from build123d import *

# Parameters (mm, degrees)
SKETCH_1_W          = 37
SKETCH_1_H          = 37
EXTRUDE_1_DEPTH     = 10.5
SKETCH_2_R          = 10
CUT_EXTRUDE_1_DEPTH = 11.5
FILLET_1_R          = 5
FILLET_2_R          = 1
SKETCH_3_R          = 1.5
CUT_EXTRUDE_2_DEPTH = 4
CUT_EXTRUDE_3_DEPTH = 8.5
CUT_EXTRUDE_4_DEPTH = 8.5
FILLET_4_R          = 0.5


with BuildPart() as part:
    # 草图1 → 凸台-拉伸1 (new body)
    with BuildSketch(Plane(origin=(0, 0, 0), x_dir=(1, 0, 0), z_dir=(0, 1, 0))):
        Rectangle(SKETCH_1_W, SKETCH_1_H)
    extrude(amount=EXTRUDE_1_DEPTH)

    # 草图2 → 切除-拉伸1 (cut, through all)
    with BuildSketch(Plane.XZ):
        Circle(SKETCH_2_R)
    extrude(amount=-CUT_EXTRUDE_1_DEPTH, mode=Mode.SUBTRACT)

    # 圆角1
    fillet_1_edges = [part.edges().sort_by_distance(p)[0] for p in [
        (-18.5, 10.5, 0),
        (0, 10.5, 18.5),
        (18.5, 10.5, 0),
        (0, 10.5, -18.5),
    ]]
    fillet(fillet_1_edges, radius=FILLET_1_R)

    # 圆角2
    fillet_2_edges = [part.edges().sort_by_distance(p)[0] for p in [
        (18.5, 2.75, -18.5),
        (18.5, 2.75, 18.5),
        (-18.5, 2.75, 18.5),
        (-18.5, 2.75, -18.5),
        (-16.730244537, 9.316480084, 16.730244537),
        (-16.730244537, 9.316480084, -16.730244537),
        (16.730244537, 9.316480084, 16.730244537),
        (16.730244537, 9.316480084, -16.730244537),
    ]]
    fillet(fillet_2_edges, radius=FILLET_2_R)

    # 草图3 → 切除-拉伸2 (cut)
    with BuildSketch(Plane.XZ):
        with Locations((15, 15)):
            Circle(SKETCH_3_R)
        with Locations((15, -15)):
            Circle(SKETCH_3_R)
        with Locations((0, -15)):
            Circle(SKETCH_3_R)
        with Locations((-15, -15)):
            Circle(SKETCH_3_R)
        with Locations((-15, 15)):
            Circle(SKETCH_3_R)
        with Locations((0, 15)):
            Circle(SKETCH_3_R)
    extrude(amount=-CUT_EXTRUDE_2_DEPTH, mode=Mode.SUBTRACT)

    # 草图4 → 切除-拉伸3 (cut)
    with BuildSketch(Plane.XZ):
        with BuildLine():
            Line((13, 12.5), (-13, 12.5))
            ThreePointArc((-13, 12.5), (-13.707106781, 12.207106781), (-14, 11.5))
            Line((-14, 11.5), (-14, -11.5))
            ThreePointArc((-14, -11.5), (-13.707106781, -12.207106781), (-13, -12.5))
            Line((-13, -12.5), (13, -12.5))
            ThreePointArc((13, -12.5), (13.707106781, -12.207106781), (14, -11.5))
            Line((14, -11.5), (14, 11.5))
            ThreePointArc((14, 11.5), (13.707106781, 12.207106781), (13, 12.5))
        make_face()
    extrude(amount=-CUT_EXTRUDE_3_DEPTH, mode=Mode.SUBTRACT)

    # 草图5 → 切除-拉伸4 (cut)
    with BuildSketch(Plane.XZ):
        with BuildLine():
            Line((-17, 12.127718677), (-17, -12.127718677))
            ThreePointArc((-17, -12.127718677), (-16.284547708, -11.744245527), (-15.5, -11.535898385))
            Line((-15.5, -11.535898385), (-15.5, 11.535898385))
            ThreePointArc((-15.5, 11.535898385), (-16.284547708, 11.744245527), (-17, 12.127718677))
        make_face()
        with BuildLine():
            Line((-12.127718677, -17), (-2.872281323, -17))
            ThreePointArc((-2.872281323, -17), (-3.455714429, -15.555011516), (-3.354101966, -14))
            Line((-3.354101966, -14), (-11.645898034, -14))
            ThreePointArc((-11.645898034, -14), (-11.544285571, -15.555011516), (-12.127718677, -17))
        make_face()
        with BuildLine():
            Line((17, -12.127718677), (17, 12.127718677))
            ThreePointArc((17, 12.127718677), (16.284547708, 11.744245527), (15.5, 11.535898385))
            Line((15.5, 11.535898385), (15.5, -11.535898385))
            ThreePointArc((15.5, -11.535898385), (16.284547708, -11.744245527), (17, -12.127718677))
        make_face()
        with BuildLine():
            Line((12.127718677, 17), (2.872281323, 17))
            ThreePointArc((2.872281323, 17), (3.455714429, 15.555011516), (3.354101966, 14))
            Line((3.354101966, 14), (11.645898034, 14))
            ThreePointArc((11.645898034, 14), (11.544285571, 15.555011516), (12.127718677, 17))
        make_face()
        with BuildLine():
            Line((-3.354101966, 14), (-11.645898034, 14))
            ThreePointArc((-11.645898034, 14), (-11.544285571, 15.555011516), (-12.127718677, 17))
            Line((-12.127718677, 17), (-2.872281323, 17))
            ThreePointArc((-2.872281323, 17), (-3.455714429, 15.555011516), (-3.354101966, 14))
        make_face()
        with BuildLine():
            Line((2.872281323, -17), (12.127718677, -17))
            ThreePointArc((12.127718677, -17), (11.544285571, -15.555011516), (11.645898034, -14))
            Line((11.645898034, -14), (3.354101966, -14))
            ThreePointArc((3.354101966, -14), (3.455714429, -15.555011516), (2.872281323, -17))
        make_face()
    extrude(amount=-CUT_EXTRUDE_4_DEPTH, mode=Mode.SUBTRACT)

    # 圆角4
    fillet_4_edges = [part.edges().sort_by_distance(p)[0] for p in [
        (-10, 10.5, 0),
    ]]
    fillet(fillet_4_edges, radius=FILLET_4_R)


solid = part.part
Verification items for the finished model (mm, model axes). A direction names the side the tool comes from. Coordinates: 2 decimals unless noted, no trailing zeros. Write each loop counter-clockwise with the first axis right and the second up, starting at its lowest first coordinate (ties: lowest second). Pieces come first, ordered by that corner, then holes. Notation, with made-up numbers: (-23.5, 5.5) - (-11.5, 5.5) arc R11 ccw to (-11.5, 22.5) - close; hole circle Ø7 at (-28.5, 33). An arc over 180 degrees is marked (long way). Answer as a JSON object with one key per item and string values.
(1) Thickness scan on line 1 along Z through (x, y) = (15, 3.2); line 2 along Z through (x, y) = (10.5, 2.5); line 3 along X through (y, z) = (1.5, -1). Record the ranges inside material, lowest first.
Report:
{"line 1": "-18.5 to -16.5, -13.5 to 13.5, 16.5 to 18.5", "line 2": "-18.5 to -17, -14 to -12.5, 12.5 to 14, 17 to 18.5", "line 3": "-18.5 to -17, -15.5 to -14, 14 to 15.5, 17 to 18.5"}
(2) Tool access check on faces 1 (the cylindrical face through (-17.07, 9, -0.24)), 2 (the flat face through (0, 4, -12.5)). Record the directions out of +Z, -Z, +X, -X, +Y, -Y that give a thin tool (end or side, any length) a straight path to the whole face; none if there is none.
Report:
{"face 1": "+Z, -Z, -X, +Y", "face 2": "-Y"}
(3) Cross-section at B-B on y = 1.5. Give the number of separate pieces and of enclosed holes in the cut face, plus the area to 3 significant figures.
Report:
{"separate pieces": "1", "enclosed holes": "13", "area": "456 mm^2"}
(4) Cross-section at A-A on z = 0. Record the cut outline in (x, y).
Report:
{"outline": "(-18.5, 0) - (-17, 0) - (-17, 8.5) - (-15.5, 8.5) - (-15.5, 0) - (-14, 0) - (-14, 8.5) - (-10, 8.5) - (-10, 10) arc R0.5 ccw to (-10.5, 10.5) - (-13.5, 10.5) arc R5 ccw to (-18.5, 5.5) - close; (10, 8.5) - (14, 8.5) - (14, 0) - (15.5, 0) - (15.5, 8.5) - (17, 8.5) - (17, 0) - (18.5, 0) - (18.5, 5.5) arc R5 ccw to (13.5, 10.5) - (10.5, 10.5) arc R0.5 ccw to (10, 10) - close"}
(5) Mould release check, pull along Z, two halves, no side actions. Record for faces 3 (the cylindrical face through (-18.215, 2.789, -18.199)), 4 (the cylindrical face through (17, 9.07, -0.24)), 5 (the cylindrical face through (11.54, 4.19, 15.53)): pulls with the +Z half, pulls with the -Z half, needs draft (parallel to the pull), parting line crosses it, or undercut.
Report:
{"face 3": "pulls with the -Z half", "face 4": "needs draft", "face 5": "undercut"}
(6) Gauge pin test, flat ends, axial feed: pin 1 Ø5 at (y, z) = (9, -4.5) entering from +X; pin 2 Ø2.5 at (x, z) = (15, -15) entering from +Y; pin 3 Ø3 at (x, z) = (-1.5, -9.5) entering from -Y; pin 4 Ø18 at (x, z) = (0, 0) entering from +Y. Record the tip position at first contact, or that the pin passes through.
Report:
{"pin 1": "x = 18.4", "pin 2": "y = 10.46", "pin 3": "y = 8.5", "pin 4": "through"}
